CAD build for the part. Positions are in the model's coordinates, mm. A direction names the side the tool comes from. Round coordinates to 2 decimals unless told otherwise and drop trailing zeros. Loops run counter-clockwise (first coordinate to the right, second up) from the corner with the lowest first, then second, coordinate; pieces in that order, holes last.
```python
from build123d import *

# Parameters (mm, degrees)
BOSS_EXTRUDE1_DEPTH     = 1
CUT_EXTRUDE1_DEPTH      = 54.925967771
CUT_EXTRUDE1_DEPTH_BACK = 54.925967771
SKETCH2_R               = 1.2


with BuildPart() as part:
    # Sketch1 → Boss-Extrude1 (new, symmetric)
    with BuildSketch(Plane(origin=(0, 0, 0), x_dir=(1, 0, 0), z_dir=(0, 1, 0))):
        Polygon((-50, 20.1), (-50, -20.1), (-24, -20.1), (-21, -17.1), (21, -17.1), (24, -20.1), (50, -20.1), (50, 20.1), (24, 20.1), (21, 17.1), (-21, 17.1), (-24, 20.1), align=None)
    extrude(amount=BOSS_EXTRUDE1_DEPTH, both=True)

    # Sketch2 → Cut-Extrude1 (cut, two sides: drawn at the far end of the back side and taken through both)
    with BuildSketch(Plane(origin=(0, 1, 0), x_dir=(1, 0, 0), z_dir=(0, 1, 0)).offset(-CUT_EXTRUDE1_DEPTH_BACK)):
        with Locations(Location((-34.95, 12.475, 0), (0, 0, 270))):
            Circle(SKETCH2_R)
        with Locations(Location((-34.95, -12.475, 0), (0, 0, 270))):
            Circle(SKETCH2_R)
        with Locations(Location((34.95, -12.475, 0), (0, 0, 270))):
            Circle(SKETCH2_R)
        with Locations(Location((34.95, 12.475, 0), (0, 0, 270))):
            Circle(SKETCH2_R)
        with BuildLine():
            Line((-18.5, 11.45), (18.5, 11.45))
            ThreePointArc((18.5, 11.45), (20.05, 9.9), (18.5, 8.35))
            Line((18.5, 8.35), (-18.5, 8.35))
            ThreePointArc((-18.5, 8.35), (-20.05, 9.9), (-18.5, 11.45))
        make_face()
        with BuildLine():
            Line((-18.5, -8.35), (18.5, -8.35))
            ThreePointArc((18.5, -8.35), (20.05, -9.9), (18.5, -11.45))
            Line((18.5, -11.45), (-18.5, -11.45))
            ThreePointArc((-18.5, -11.45), (-20.05, -9.9), (-18.5, -8.35))
        make_face()
    extrude(amount=CUT_EXTRUDE1_DEPTH + CUT_EXTRUDE1_DEPTH_BACK, mode=Mode.SUBTRACT)


solid = part.part
```
Item 1: Probe line 1 (Z direction, x = -35, y = -0.3); line 2 (Z direction, x = 5, y = -0.05); line 3 (X direction, y = -0.45, z = 12). List the from-to ranges inside material, lowest first.
Answers follow:
line 1: z = -20.1 to -13.67, -11.28 to 11.28, 13.67 to 20.1
line 2: z = -17.1 to -11.45, -8.35 to 8.35, 11.45 to 17.1
line 3: x = -50 to -36.05, -33.85 to 33.85, 36.05 to 50
Item 2: Cut at C-C, the plane x = 10.5. Give the cut face in (y, z).
Answers follow:
outline: (-1, -17.1) - (1, -17.1) - (1, -11.45) - (-1, -11.45) - close; (-1, -8.35) - (1, -8.35) - (1, 8.35) - (-1, 8.35) - close; (-1, 11.45) - (1, 11.45) - (1, 17.1) - (-1, 17.1) - close
Item 3: Two-plate mould, pull along Z, no slides. Class faces 6 (the flat face through (0, 0, -17.1)), 7 (the flat face through (-22.5, 0, 18.6)), 8 (the cylindrical face through (-20.05, -0.01, 9.93)): released by +Z, released by -Z, zero draft, split by the parting line, or undercut.
Answers follow:
face 6: released by -Z
face 7: released by +Z
face 8: undercut
Item 4: 3-axis set-ups, long thin cutter, end or side, ignore diameter. For faces 1 (the flat face through (0, 0, 8.35)), 2 (the flat face through (0, 0, 17.1)), 3 (the flat face through (-1, 1, 0)), 4 (the flat face through (-22.5, 0, -18.6)), 5 (the flat face through (50, 0, 0)): which of +Z, -Z, +X, -X, +Y, -Y reach the whole face in a straight line?
Answers follow:
face 1: +Y, -Y
face 2: +Z, +Y, -Y
face 3: +Z, -Z, +X, -X, +Y
face 4: -Z, +Y, -Y
face 5: +Z, -Z, +X, +Y, -Y
Item 5: Cut at A-A, the plane y = 0.05. Give the cut face in (x, z) (3 decimals), plus the area to 3 significant figures.
Answers follow:
outline: (-50, -20.1) - (-24, -20.1) - (-21, -17.1) - (21, -17.1) - (24, -20.1) - (50, -20.1) - (50, 20.1) - (24, 20.1) - (21, 17.1) - (-21, 17.1) - (-24, 20.1) - (-50, 20.1) - close; hole circle Ø2.4 at (-34.95, -12.475); hole circle Ø2.4 at (-34.95, 12.475); hole (-18.5, -11.45) - (18.5, -11.45) arc R1.55 ccw to (18.5, -8.35) - (-18.5, -8.35) arc R1.55 ccw to start; hole (-18.5, 8.35) - (18.5, 8.35) arc R1.55 ccw to (18.5, 11.45) - (-18.5, 11.45) arc R1.55 ccw to start; hole circle Ø2.4 at (34.95, -12.475); hole circle Ø2.4 at (34.95, 12.475)
area: 3,490 mm2
Item 6: Cut at B-B, the plane z = -9.9. Give the cut face in (x, y), plus the area to 3 significant figures.
Answers follow:
outline: (-50, -1) - (-20.05, -1) - (-20.05, 1) - (-50, 1) - close; (20.05, -1) - (50, -1) - (50, 1) - (20.05, 1) - close
area: 120 mm2
Item 7: Flat gauge pins, fed straight in: P1, Ø0.6, axis at x = -3, y = 0, coming from the -Z side; P2, Ø1, axis at x = -1, y = 0, coming from the +Z side. Where does each tip first touch, or does it go through?
Answers follow:
P1: stops at z = -17.1
P2: stops at z = 17.1
